from build123d import *

# Parameters (mm, degrees)
BOSS_EXTRUDE1_DEPTH = 20
SKETCH2_R           = 146.05
CUT_EXTRUDE1_DEPTH  = 5
CUT_EXTRUDE2_REACH  = 235.968
SKETCH3_R           = 101.6
CUT_EXTRUDE3_REACH  = 236.342
SKETCH4_W           = 42
SKETCH4_H           = 42
CUT_EXTRUDE4_REACH  = 236.342
SKETCH5_R           = 2.75


with BuildPart() as part:
    # Sketch1 → Boss-Extrude1 (new body)
    with BuildSketch(Plane(origin=(0, 0, 0), x_dir=(1, 0, 0), z_dir=(0, 1, 0))):
        with BuildLine():
            Line((165.1, 0), (165.1, -165.1))
            Line((165.1, -165.1), (-165.1, -165.1))
            Line((-165.1, -165.1), (-165.1, 165.1))
            Line((-165.1, 165.1), (0, 165.1))
            ThreePointArc((0, 165.1), (116.743329574, 116.743329574), (165.1, 0))
        make_face()
    extrude(amount=BOSS_EXTRUDE1_DEPTH)

    # Sketch2 → Cut-Extrude1 (cut)
    with BuildSketch(Plane(origin=(0, 20, 0), x_dir=(1, 0, 0), z_dir=(0, 1, 0))):
        with Locations(Location((0, 0, 0), (0, 0, 270))):
            Circle(SKETCH2_R)
    extrude(amount=-CUT_EXTRUDE1_DEPTH, mode=Mode.SUBTRACT)

    # Sketch3 → Cut-Extrude2 (cut, up to next)
    with BuildSketch(Plane(origin=(0, 15, 0), x_dir=(1, 0, 0), z_dir=(0, 1, 0)), mode=Mode.PRIVATE) as cut_extrude2_sk1:
        with Locations(Location((0, 0, 0), (0, 0, 270))):
            Circle(SKETCH3_R)
    cut_extrude2_tool1 = extrude(cut_extrude2_sk1.sketch, amount=-CUT_EXTRUDE2_REACH, mode=Mode.PRIVATE) & part.part
    add(cut_extrude2_tool1.solids().sort_by_distance((0, 15, 0))[0], mode=Mode.SUBTRACT)

    # Sketch4 → Cut-Extrude3 (cut, up to next)
    with BuildSketch(Plane(origin=(0, 20, 0), x_dir=(1, 0, 0), z_dir=(0, 1, 0)), mode=Mode.PRIVATE) as cut_extrude3_sk1:
        with Locations((-144.1, -144.1)):
            Rectangle(SKETCH4_W, SKETCH4_H)
    cut_extrude3_tool1 = extrude(cut_extrude3_sk1.sketch, amount=-CUT_EXTRUDE3_REACH, mode=Mode.PRIVATE) & part.part
    add(cut_extrude3_tool1.solids().sort_by_distance((-144.1, 20, 144.1))[0], mode=Mode.SUBTRACT)

    # Sketch5 → Cut-Extrude4 (cut, up to next)
    with BuildSketch(Plane(origin=(0, 20, 0), x_dir=(1, 0, 0), z_dir=(0, 1, 0)), mode=Mode.PRIVATE) as cut_extrude4_sk1:
        with Locations(Location((-103.1, -135.1, 0), (0, 0, 270))):
            Circle(SKETCH5_R)
    cut_extrude4_tool1 = extrude(cut_extrude4_sk1.sketch, amount=-CUT_EXTRUDE4_REACH, mode=Mode.PRIVATE) & part.part
    # Sketch5 → Cut-Extrude4 (cut, up to next)
    with BuildSketch(Plane(origin=(0, 20, 0), x_dir=(1, 0, 0), z_dir=(0, 1, 0)), mode=Mode.PRIVATE) as cut_extrude4_sk2:
        with Locations(Location((145.1, -135.1, 0), (0, 0, 270))):
            Circle(SKETCH5_R)
    cut_extrude4_tool2 = extrude(cut_extrude4_sk2.sketch, amount=-CUT_EXTRUDE4_REACH, mode=Mode.PRIVATE) & part.part
    # Sketch5 → Cut-Extrude4 (cut, up to next)
    with BuildSketch(Plane(origin=(0, 20, 0), x_dir=(1, 0, 0), z_dir=(0, 1, 0)), mode=Mode.PRIVATE) as cut_extrude4_sk3:
        with Locations(Location((-103.1, -155.1, 0), (0, 0, 270))):
            Circle(SKETCH5_R)
    cut_extrude4_tool3 = extrude(cut_extrude4_sk3.sketch, amount=-CUT_EXTRUDE4_REACH, mode=Mode.PRIVATE) & part.part
    # Sketch5 → Cut-Extrude4 (cut, up to next)
    with BuildSketch(Plane(origin=(0, 20, 0), x_dir=(1, 0, 0), z_dir=(0, 1, 0)), mode=Mode.PRIVATE) as cut_extrude4_sk4:
        with Locations(Location((145.1, -155.1, 0), (0, 0, 270))):
            Circle(SKETCH5_R)
    cut_extrude4_tool4 = extrude(cut_extrude4_sk4.sketch, amount=-CUT_EXTRUDE4_REACH, mode=Mode.PRIVATE) & part.part
    # Sketch5 → Cut-Extrude4 (cut, up to next)
    with BuildSketch(Plane(origin=(0, 20, 0), x_dir=(1, 0, 0), z_dir=(0, 1, 0)), mode=Mode.PRIVATE) as cut_extrude4_sk5:
        with Locations(Location((-155.1, 145.1, 0), (0, 0, 270))):
            Circle(SKETCH5_R)
    cut_extrude4_tool5 = extrude(cut_extrude4_sk5.sketch, amount=-CUT_EXTRUDE4_REACH, mode=Mode.PRIVATE) & part.part
    # Sketch5 → Cut-Extrude4 (cut, up to next)
    with BuildSketch(Plane(origin=(0, 20, 0), x_dir=(1, 0, 0), z_dir=(0, 1, 0)), mode=Mode.PRIVATE) as cut_extrude4_sk6:
        with Locations(Location((-155.1, -103.1, 0), (0, 0, 270))):
            Circle(SKETCH5_R)
    cut_extrude4_tool6 = extrude(cut_extrude4_sk6.sketch, amount=-CUT_EXTRUDE4_REACH, mode=Mode.PRIVATE) & part.part
    # Sketch5 → Cut-Extrude4 (cut, up to next)
    with BuildSketch(Plane(origin=(0, 20, 0), x_dir=(1, 0, 0), z_dir=(0, 1, 0)), mode=Mode.PRIVATE) as cut_extrude4_sk7:
        with Locations(Location((-135.1, 145.1, 0), (0, 0, 270))):
            Circle(SKETCH5_R)
    cut_extrude4_tool7 = extrude(cut_extrude4_sk7.sketch, amount=-CUT_EXTRUDE4_REACH, mode=Mode.PRIVATE) & part.part
    # Sketch5 → Cut-Extrude4 (cut, up to next)
    with BuildSketch(Plane(origin=(0, 20, 0), x_dir=(1, 0, 0), z_dir=(0, 1, 0)), mode=Mode.PRIVATE) as cut_extrude4_sk8:
        with Locations(Location((-135.1, -103.1, 0), (0, 0, 270))):
            Circle(SKETCH5_R)
    cut_extrude4_tool8 = extrude(cut_extrude4_sk8.sketch, amount=-CUT_EXTRUDE4_REACH, mode=Mode.PRIVATE) & part.part
    add(cut_extrude4_tool1.solids().sort_by_distance((-103.1, 20, 135.1))[0], mode=Mode.SUBTRACT)
    add(cut_extrude4_tool2.solids().sort_by_distance((145.1, 20, 135.1))[0], mode=Mode.SUBTRACT)
    add(cut_extrude4_tool3.solids().sort_by_distance((-103.1, 20, 155.1))[0], mode=Mode.SUBTRACT)
    add(cut_extrude4_tool4.solids().sort_by_distance((145.1, 20, 155.1))[0], mode=Mode.SUBTRACT)
    add(cut_extrude4_tool5.solids().sort_by_distance((-155.1, 20, -145.1))[0], mode=Mode.SUBTRACT)
    add(cut_extrude4_tool6.solids().sort_by_distance((-155.1, 20, 103.1))[0], mode=Mode.SUBTRACT)
    add(cut_extrude4_tool7.solids().sort_by_distance((-135.1, 20, -145.1))[0], mode=Mode.SUBTRACT)
    add(cut_extrude4_tool8.solids().sort_by_distance((-135.1, 20, 103.1))[0], mode=Mode.SUBTRACT)


solid = part.part
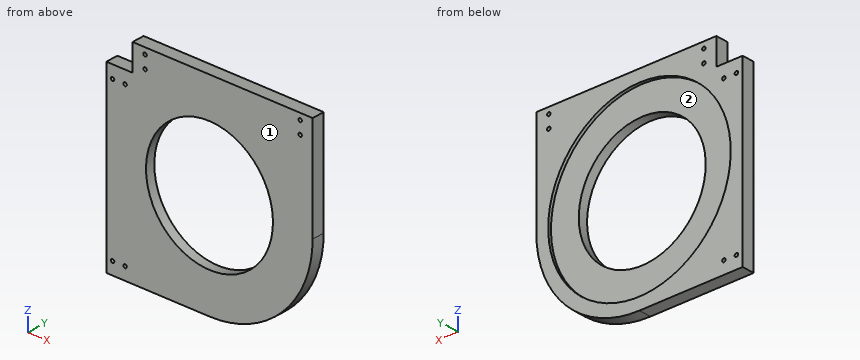
Check sheet for the modelled part. Datum: model origin and axes. Units: mm. Face numbers are marked on the shaded views. Coordinates: 2 decimals unless noted, no trailing zeros. Loops run counter-clockwise (first coordinate to the right, second up) from the corner with the lowest first, then second, coordinate; pieces in that order, holes last. Notation, with made-up numbers: (86, 29) -> (132, 29) arc R15 cw to (132, 43) -> close; hole circle Ø10 at (-16, 76.25). An arc over 180 degrees is marked (long way). Write item = value, one per line. Start each with the question number.
1. Section check A-A on z = 84. Record the cut outline in (x, y).
2. Section check B-B on x = 62.5. Record the cut outline in (y, z).
3. Section check C-C on y = 6.5. Give the number of separate pieces and of enclosed holes in the cut face, then the cut area to 3 significant figures.
4. Draft check along Z on the marked faces 1 and 2. Enter one of: released by +Z, released by -Z, zero draft, split by the parting line, or undercut.
5. Section check D-D on x = 123.5. Record the cut outline in (y, z), then the cut area to 3 significant figures.
6. Depth check by flat-ended pin: P1, Ø3.5, axis at x = -155.1, z = -145.1, coming from the -Y side; P2, Ø6.5, axis at x = -135.1, z = -145.1, coming from the -Y side; P3, Ø2, axis at y = 13.5, z = -72.5, coming from the +X side; P4, Ø10, axis at y = 5.5, z = 134, coming from the -X side. Enter the tip coordinate at first touch or a pass-through.
7. Material ranges on line 1 (X direction, y = 15.75, z = 155.1); line 2 (Z direction, x = -155.1, y = 14); line 3 (X direction, y = 11.5, z = 103), recorded low to high.
Responses:
q1.outline = (-165.1, 0) -> (-57.15, 0) -> (-57.15, 15) -> (-119.48, 15) -> (-119.48, 20) -> (-165.1, 20) -> close; (57.15, 0) -> (165.1, 0) -> (165.1, 20) -> (119.48, 20) -> (119.48, 15) -> (57.15, 15) -> close
q2.outline = (0, -152.81) -> (20, -152.81) -> (20, -132) -> (15, -132) -> (15, -80.1) -> (0, -80.1) -> close; (0, 80.1) -> (15, 80.1) -> (15, 132) -> (20, 132) -> (20, 165.1) -> (0, 165.1) -> close
q3.separate_pieces = 1
q3.enclosed_holes = 9
q3.area = 68,800 mm2
q4.face_1 = zero draft
q4.face_2 = undercut
q5.outline = (0, -109.57) -> (20, -109.57) -> (20, -77.96) -> (15, -77.96) -> (15, 77.96) -> (20, 77.96) -> (20, 165.1) -> (0, 165.1) -> close
q5.area = 4,710 mm2
q6.P1 = through
q6.P2 = 0
q6.P3 = 148.81
q6.P4 = -123.1
q7.line_1 = -123.1 to -105.85, -100.35 to 142.35, 147.85 to 165.1
q7.line_2 = -165.1 to -147.85, -142.35 to 100.35, 105.85 to 123.1
q7.line_3 = -165.1 to -157.85, -152.35 to -137.85, -132.35 to 165.1
